from build123d import *

# Parameters (mm, degrees)
SKETCH1_R           = 12.5
SKETCH1_W           = 175
SKETCH1_H           = 15
BOSS_EXTRUDE1_DEPTH = 30
CUT_EXTRUDE2_REACH  = 180.185
SKETCH2_R           = 2.5
SKETCH2_3_R         = 6
SKETCH2_3_R_2       = 2.5
CUT_EXTRUDE3_DEPTH  = 4
SKETCH3_W           = 175
SKETCH3_H           = 10
CUT_EXTRUDE4_DEPTH  = 5


with BuildPart() as part:
    # Sketch1 → Boss-Extrude1 (new body)
    with BuildSketch(Plane.XY):
        with Locations((162.5, 0)):
            Circle(SKETCH1_R)
        with Locations((87.5, 0)):
            Circle(SKETCH1_R)
        with Locations((87.5, 7.5)):
            Rectangle(SKETCH1_W, SKETCH1_H)
        with BuildLine():
            ThreePointArc((175, 0), (162.5, 12.5), (150, 0))
            Line((150, 0), (162.5, 0))
            Line((162.5, 0), (175, 0))
        make_face()
        with BuildLine():
            Line((162.5, 0), (150, 0))
            ThreePointArc((150, 0), (162.5, -12.5), (175, 0))
            Line((175, 0), (162.5, 0))
        make_face()
        with BuildLine():
            ThreePointArc((100, 0), (87.5, 12.5), (75, 0))
            Line((75, 0), (87.5, 0))
            Line((87.5, 0), (100, 0))
        make_face()
        with BuildLine():
            Line((87.5, 0), (75, 0))
            ThreePointArc((75, 0), (87.5, -12.5), (100, 0))
            Line((100, 0), (87.5, 0))
        make_face()
    extrude(amount=BOSS_EXTRUDE1_DEPTH)

    # Sketch2 → Cut-Extrude2 (cut, up to next)
    with BuildSketch(Plane.XY.offset(30), mode=Mode.PRIVATE) as cut_extrude2_sk1:
        with Locations((87.5, 0)):
            Circle(SKETCH2_R)
    cut_extrude2_tool1 = extrude(cut_extrude2_sk1.sketch, amount=-CUT_EXTRUDE2_REACH, mode=Mode.PRIVATE) & part.part
    # Sketch2 → Cut-Extrude2 (cut, up to next)
    with BuildSketch(Plane.XY.offset(30), mode=Mode.PRIVATE) as cut_extrude2_sk2:
        with Locations((162.5, 0)):
            Circle(SKETCH2_R)
    cut_extrude2_tool2 = extrude(cut_extrude2_sk2.sketch, amount=-CUT_EXTRUDE2_REACH, mode=Mode.PRIVATE) & part.part
    add(cut_extrude2_tool1.solids().sort_by_distance((87.5, 0, 30))[0], mode=Mode.SUBTRACT)
    add(cut_extrude2_tool2.solids().sort_by_distance((162.5, 0, 30))[0], mode=Mode.SUBTRACT)

    # Sketch2_3 → Cut-Extrude3 (cut)
    # profile 1 of 2: a face of its own
    with BuildSketch(Plane.XY.offset(30)):
        with Locations((87.5, 0)):
            Circle(SKETCH2_3_R)
        with Locations((87.5, 0)):
            Circle(SKETCH2_3_R_2, mode=Mode.SUBTRACT)
    # profile 2 of 2: a face of its own
    with BuildSketch(Plane.XY.offset(30)):
        with Locations((162.5, 0)):
            Circle(SKETCH2_3_R)
        with Locations((162.5, 0)):
            Circle(SKETCH2_3_R_2, mode=Mode.SUBTRACT)
    extrude(amount=-CUT_EXTRUDE3_DEPTH, mode=Mode.SUBTRACT)

    # Sketch3 → Cut-Extrude4 (cut)
    with BuildSketch(Plane(origin=(0, 15, 0), x_dir=(1, 0, 0), z_dir=(0, 1, 0))):
        with Locations((87.5, -15)):
            Rectangle(SKETCH3_W, SKETCH3_H)
    extrude(amount=-CUT_EXTRUDE4_DEPTH, mode=Mode.SUBTRACT)


solid = part.part
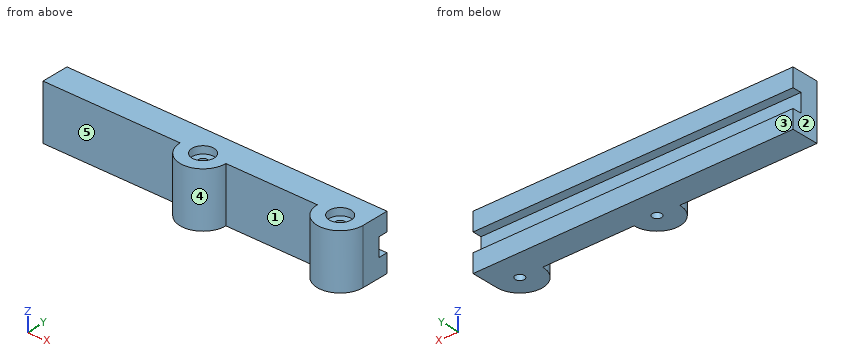
The model under review builds one solid part; all positions refer to its coordinate system, in mm. Face numbers are marked on the shaded views. A direction names the side the tool comes from. Round coordinates to 2 decimals unless told otherwise and drop trailing zeros. Loops run counter-clockwise (first coordinate to the right, second up) from the corner with the lowest first, then second, coordinate; pieces in that order, holes last. Notation, with made-up numbers: (19.5, -9.75) -> (71.5, -9.75) arc R19 ccw to (71.5, 0.25) -> close; hole circle Ø8 at (61, 32.25). An arc over 180 degrees is marked (long way). One line per question, with ' | ' between items. Start each with the question number.
Item 1: Draft analysis for pull direction X (two halves, no side actions). For the marked faces 1, 2 and 3, state which applies: +X half, -X half, draft (parallel to the pull), parting line (faces both ways), or undercut.
Item 2: For pin 1 (15 mm diameter, centred on x = 136, z = 16, fed in from -Y); pin 2 (12 mm diameter, centred on y = -9, z = 8.5, fed in from -X); pin 3 (8 mm diameter, centred on y = -9.5, z = 3.5, fed in from -X) (3 decimals), all flat-tipped, find the tip position at first contact; note any pin that passes through.
Item 3: Add section B-B, the plane y = 12. Write out the cut boundary in (x, z), then the cut area to 3 significant figures.
Item 4: Wall thickness on line 1 along Y through (x, z) = (87.5, 15.5); line 2 along X through (y, z) = (5, 28.5); line 3 along X through (y, z) = (-5, 9.25): over which ranges is each line inside the solid? List them lowest first. Write a range as [from, to].
Item 5: Add section D-D, the plane x = 126. Write out the cut boundary in (y, z), then the cut area to 3 significant figures.
Item 6: Machinability: for the marked faces 4 and 5, which of the approach directions +Z, -Z, +X, -X, +Y, -Y give a long, thin tool a straight path to every point of the face, cutting with its end or side? Answer none if there is none.
Item 7: Add section A-A, the plane z = 2.5. Write out the cut boundary in (x, y).
Item 8: Add section C-C, the plane x = 162.5. Write out the cut boundary in (y, z).
Return value:
1) face 1: undercut | face 2: -X half | face 3: draft
2) pin 1: stops at y = 0 | pin 2: stops at x = 75.37 | pin 3: stops at x = 76.275
3) outline: (0, 0) -> (175, 0) -> (175, 10) -> (0, 10) -> close; (0, 20) -> (175, 20) -> (175, 30) -> (0, 30) -> close | area: 3,500 mm2
4) line 1: y = [-12.5, -2.5], [2.5, 10] | line 2: x = [0, 84.18], [90.82, 159.18], [165.82, 175] | line 3: x = [76.04, 98.96], [151.04, 173.96]
5) outline: (0, 0) -> (15, 0) -> (15, 10) -> (10, 10) -> (10, 20) -> (15, 20) -> (15, 30) -> (0, 30) -> close | area: 400 mm2
6) face 4: +Z, -Z, -Y | face 5: +Z, -Z, -X, -Y
7) outline: (0, 0) -> (75, 0) arc R12.5 ccw to (100, 0) -> (150, 0) arc R12.5 ccw to (175, 0) -> (175, 15) -> (0, 15) -> close; hole circle Ø5 at (87.5, 0); hole circle Ø5 at (162.5, 0)
8) outline: (-12.5, 0) -> (-2.5, 0) -> (-2.5, 26) -> (-6, 26) -> (-6, 30) -> (-12.5, 30) -> close; (2.5, 0) -> (15, 0) -> (15, 10) -> (10, 10) -> (10, 20) -> (15, 20) -> (15, 30) -> (6, 30) -> (6, 26) -> (2.5, 26) -> close
